Autodesk Inventor part; units mm, degrees
ref_plane "YZ Plane" through (0, 0, 0) normal (1, 0, 0) x (0, 1, 0)
ref_plane "XZ Plane" through (0, 0, 0) normal (0, 1, 0) x (-1, 0, 0)
ref_plane "XY Plane" through (0, 0, 0) normal (0, 0, 1) x (1, 0, 0)
sketch "Boceto1" plane through (0, 0, 0) normal (0, 1, 0) x (-1, 0, 0)
  line L0 (0, 0) -> (0, -150)
  line L1 (0, -150) -> (-150, -150)
  line L2 (-150, -150) -> (-150, 0)
  line L3 (-150, 0) -> (0, 0)
extrude "Extrusión1" add sketch "Boceto1" along normal blind 4
sketch "Boceto2" plane through (0, 4, 0) normal (0, 1, 0) x (1, 0, 0)
  line L0 (0, 0) -> (150, 0)
  circle A0 centre (103.5, 67.5) radius 12.5
extrude "Extrusión2" cut sketch "Boceto2" against normal blind 1
sketch "Boceto3" plane through (0, 4, 0) normal (0, 1, 0) x (1, 0, 0)
  circle A0 centre (103.5, 67.5) radius 12.5
  circle A1 centre (103.5, 76) radius 1.5
  circle A2 centre (103.5, 59) radius 1.5
  circle A3 centre (103.5, 67.5) radius 3.5
  point P0 (0, 0)
extrude "Extrusión3" cut sketch "Boceto3" against normal blind 4 contours A1 | A2 | A3
sketch "Boceto4" plane through (0, 0, 0) normal (0, -1, 0) x (1, 0, 0)
  point P0 (0, 0)
sketch "Boceto5" plane through (0, 0, 0) normal (0, -1, 0) x (1, 0, 0)
  line L0 (0, 0) -> (0, -4)
  line L1 (150, -4) -> (150, 0)
  line L2 (150, 0) -> (0, 0)
  line L3 (4, -4) -> (146, -4)
  line L4 (0, 0) -> (4, 0)
  line L5 (0, 0) -> (150, 0)
  line L6 (4, -4) -> (4, -146)
  line L7 (0, -150) -> (0, 0)
  line L8 (0, -4) -> (0, -150)
  line L9 (0, -150) -> (150, -150)
  line L10 (150, -150) -> (150, -4)
  line L11 (0, -150) -> (0, -146)
  line L12 (4, -146) -> (146, -146)
  line L13 (150, -150) -> (146, -150)
  line L14 (150, -150) -> (0, -150)
  line L15 (146, -146) -> (146, -4)
extrude "Extrusión4" add sketch "Boceto5" along normal blind 46
sketch "Boceto6" plane through (0, -46, 0) normal (0, -1, 0) x (1, 0, 0)
  line L0 (4, -4) -> (4, -146)
  line L1 (4, -146) -> (146, -146)
  line L2 (4, -146) -> (146, -146)
  line L3 (146, -146) -> (146, -4)
  line L4 (146, -4) -> (4, -4)
  line L5 (1.7, -4) -> (1.7, -148.3)
  line L6 (1.7, -148.3) -> (148.3, -148.3)
  line L7 (150, -150) -> (0, -150)
  line L8 (146, -1.7) -> (1.7, -1.7)
  line L9 (1.7, -4) -> (1.7, -1.7)
  line L10 (146, -1.7) -> (148.3, -1.7)
  line L11 (148.3, -1.7) -> (148.3, -148.3)
  point P0 (0, 0)
extrude "Extrusión5" cut sketch "Boceto6" against normal blind 10
sketch "Boceto7" plane through (0, -36, 0) normal (0, -1, 0) x (1, 0, 0)
  point P0 (0, 0)
sketch "Boceto8" plane through (4, 0, -4) normal (1, 0, 0) x (0, 0, -1)
  point P0 (-4, 0)
sketch "Boceto9" plane through (0, 4, -150) normal (-1, 0, 0) x (0, 0, 1)
  line L0 (150, -50) -> (146, -50)
  line L1 (150, -50) -> (150, 0)
  line L2 (150, 0) -> (0, 0)
  line L3 (150, -50) -> (0, -50)
  line L4 (0, 0) -> (0, -50)
  line L5 (0, -50) -> (4, -50)
  line L6 (0, 0) -> (0, -4)
  line L7 (4, 0) -> (146, 0)
  line L8 (150, 0) -> (146, 0)
  line L9 (0, 0) -> (150, 0)
  line L10 (146, 0) -> (146, -50)
  line L11 (0, 0) -> (4, 0)
  line L12 (4, 0) -> (4, -50)
  line L13 (4, -50) -> (146, -50)
  point P0 (150, -4)
extrude "Extrusión6" cut sketch "Boceto9" against normal blind 4 contours L3 L12 L2 L10
sketch "Boceto10" plane through (0, 4, 0) normal (0, 0, 1) x (1, 0, 0)
  point P0 (0, -4)
sketch "Boceto11" plane through (4, 4, -150) normal (-1, 0, 0) x (0, 0, 1)
  line L0 (146, -4) -> (4, -4)
  line L1 (146, -4) -> (146, -40)
  line L2 (4, -4) -> (146, -4)
  line L3 (146, 0) -> (150, 0)
  line L4 (146, -4) -> (146, 0)
  line L5 (146, 0) -> (4, 0)
  line L6 (4, 0) -> (4, -4)
  point P0 (150, -4)
extrude "Extrusión7" add sketch "Boceto11" along normal blind 4
sketch "Boceto12" plane through (0, 4, 0) normal (0, 0, 1) x (1, 0, 0)
  point P0 (0, -4)
properties part number "base sup"
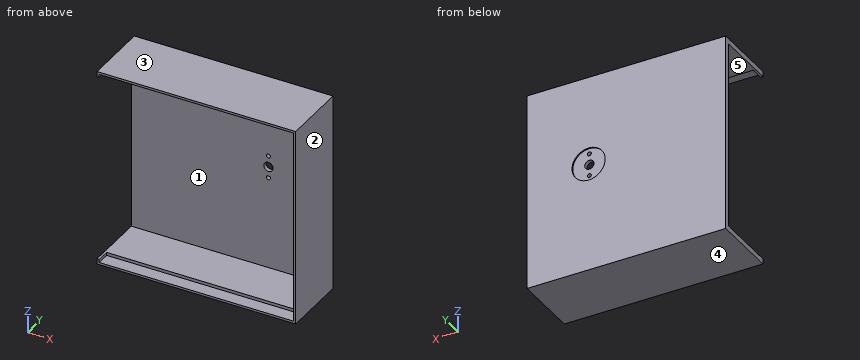
Can you work these out from the model? Positions are in its coordinate system, mm. Face numbers are marked on the shaded views. A direction names the side the tool comes from. Coordinates: 2 decimals unless noted, no trailing zeros. Write each loop counter-clockwise with the first axis right and the second up, starting at its lowest first coordinate (ties: lowest second). Pieces come first, ordered by that corner, then holes.
Q1. Imagine slicing it at C-C, the plane z = -26.5. List the corners of the cut face in (x, y) for me, plus the area to 3 significant figures.
Results found:
outline: (0, 0) - (146, 0) - (146, -36) - (148.3, -36) - (148.3, -46) - (150, -46) - (150, 4) - (0, 4) - close
area: 761 mm2
Q2. Imagine slicing it at A-A, the plane x = 14. List the corners of the cut face in (y, z) for me.
Results found:
outline: (-46, -150) - (4, -150) - (4, 0) - (-46, 0) - (-46, -1.7) - (-36, -1.7) - (-36, -4) - (0, -4) - (0, -146) - (-36, -146) - (-36, -148.3) - (-46, -148.3) - close
Q3. Imagine slicing it at B-B, the plane z = -67.5. List the corners of the cut face in (x, y) for me, plus the area to 3 significant figures.
Results found:
outline: (0, 0) - (100, 0) - (100, 3) - (91, 3) - (91, 4) - (0, 4) - close; (107, 0) - (146, 0) - (146, -36) - (148.3, -36) - (148.3, -46) - (150, -46) - (150, 4) - (116, 4) - (116, 3) - (107, 3) - close
area: 715 mm2
Q4. Imagine slicing it at D-D, the plane y = -41.5. List the corners of the cut face in (x, z) for me.
Results found:
outline: (0, -150) - (150, -150) - (150, 0) - (0, 0) - (0, -4) - (1.7, -4) - (1.7, -1.7) - (148.3, -1.7) - (148.3, -148.3) - (1.7, -148.3) - (1.7, -146) - (0, -146) - close
Q5. Please list where these lines run through material, in increasing order: L1, parallel to Z at x = 103.5, y = 0.8; L2, parallel to Z at x = 98, y = -32; L3, parallel to X at y = 2, z = -59.
Results found:
L1: z = -150 to -77.5, -74.5 to -71, -64 to -60.5, -57.5 to 0
L2: z = -150 to -146, -4 to 0
L3: x = 0 to 102, 105 to 150
Q6. If we mould it in two halves opening along Z, with no side actions, what happens to the marked faces 1, 2 and 3? For each: +Z half, -Z half, draft (parallel to the pull), parting line (faces both ways), or undercut.
Results found:
face 1: undercut
face 2: draft
face 3: +Z half
Q7. Which directions (+Z, -Z, +X, -X, +Y, -Y) give clear straight access to the entire face, cutting with the end or side of a thin tool? Please do the marked faces 4 and 5.
Results found:
face 4: -Z, +X, -X, +Y, -Y
face 5: -X, -Y
Q8. For P1, Ø22.5, axis at x = 103.5, z = -67.5, coming from the -Y side; P2, Ø11, axis at y = -18, z = -92.5, coming from the -X side, each with a flat end and sliding along its axis, tell me the tip position at first contact or that it passes through.
Results found:
P1: stops at y = 0
P2: stops at x = 146
